Part model, mm, in its own coordinate system. Round coordinates to 2 decimals unless told otherwise and drop trailing zeros. Order: outer loops, then holes, each group sorted by start corner. A loop starts at its lowest first (then second) coordinate and runs counter-clockwise, first axis right, second up. Notation, with made-up numbers: (61, 69.5) -> (71, 69.5) arc R22 ccw to (71, 98.5) -> close; hole circle Ø1 at (-27, 5). An arc over 180 degrees is marked (long way). Answer as a JSON object with one key per item and string values. Group by question number.
Autodesk Inventor part; units mm, degrees
ref_plane "YZ Plane" through (0, 0, 0) normal (1, 0, 0) x (0, 1, 0)
ref_plane "XZ Plane" through (0, 0, 0) normal (0, 1, 0) x (-1, 0, 0)
ref_plane "XY Plane" through (0, 0, 0) normal (0, 0, 1) x (1, 0, 0)
sketch "Skizze1" plane through (0, 0, 0) normal (0, 0, 1) x (1, 0, 0)
  line L0 (-110, -65) -> (110, -65)
  line L1 (110, -65) -> (110, 65)
  line L2 (110, 65) -> (-110, 65)
  line L3 (-110, 65) -> (-110, -65)
  line L4 (-110, -65) -> (110, 65) construction
  line L5 (110, -65) -> (-110, 65) construction
  point P0 (0, 0)
  dimension "d0" = 220
  dimension "d1" = 130
extrude "Grundkörper" add sketch "Skizze1" along normal blind 5
sketch "Skizze2" plane through (0, 0, 5) normal (0, 0, 1) x (1, 0, 0)
  line L0 (110, 65) -> (-110, 65) construction
  line L1 (-110, 65) -> (-110, -65) construction
  line L2 (110, -65) -> (110, 65) construction
  line L3 (-110, -65) -> (110, -65) construction
  line L4 (-95, -50) -> (95, -50) construction
  line L5 (95, -50) -> (95, 50) construction
  line L6 (95, 50) -> (-95, 50) construction
  line L7 (-95, 50) -> (-95, -50) construction
  line L8 (-95, -50) -> (95, 50) construction
  line L9 (95, -50) -> (-95, 50) construction
  line L10 (0, 65) -> (0, -65) construction
  point P0 (0, 0)
  point P1 (0, 50)
  point P2 (-95, 16.6667)
  point P3 (-95, -16.6667)
  point P4 (-95, -50)
  point P5 (0, 50)
  point P6 (0, 16.6667)
  point P7 (0, -16.6667)
  point P8 (0, -50)
  point P9 (-47.5, 50)
  point P10 (-47.5, -50)
  point P11 (0, 50)
  point P12 (0, -50)
  point P13 (95, 50)
  point P14 (95, 16.6667)
  point P15 (95, -16.6667)
  point P16 (95, -50)
  point P17 (95, -50)
  point P18 (47.5, 50)
  point P19 (47.5, -50)
  dimension "d4" = 15
  dimension "d5" = 15
  dimension "d6" = 100
  dimension "d7" = 190
  dimension "d17" = 33.3333
  dimension "d20" = 95
  dimension "d25" = 47.5
hole "Boh_M6" at (-95, 50, 5) at (0, 50, 5) at (-95, 16.6667, 5) at (-95, -16.6667, 5) at (-95, -50, 5) at (-95, -50, 5) at (0, 16.6667, 5) at (0, -16.6667, 5) at (0, -50, 5) at (-47.5, 50, 5) at (-47.5, -50, 5) at (47.5, 50, 5) at (95, 50, 5) at (95, 16.6667, 5) at (95, -16.6667, 5) at (95, -50, 5) at (95, -50, 5) at (47.5, -50, 5) direction (0, 0, -1) diameter 6.6 end through all
equation "\"d0\" = Chassis_Width"
equation "\"Chassis_Width\" = 220"
equation "\"Rocker_Screw_Distance\" = 32.5"
equation "\"Rocker_Screw_Distance_Bottom\" = 76"
properties part number "100-10-FRAME-DIFFERENTIAL-REINF-01" material "Aluminium 6061"
Q1. Band-saw the part on A-A (x = -95). List the corners of the cut face in (y, z), plus the area to 3 significant figures.
Q2. Wall check: line 1 (X direction, y = -50, z = 2.45); line 2 (Y direction, x = -47.5, z = 3.2); line 3 (Y direction, x = -95, z = 1.25). Give the ranges that are in metal, low to high. Write a range as [from, to].
Q3. Two-plate mould, pull along Y, no slides. Class faces 1 (the flat face through (-2, -65, 2)), 2 (the flat face through (-2, 1, 5)), 3 (the cylindrical face through (-97.23, 52.43, 2.46)): +Y half, -Y half, draft (parallel to the pull), parting line (faces both ways), or undercut.
Q4. Band-saw the part on D-D (x = 47.5). List the corners of the cut face in (y, z), plus the area to 3 significant figures.
Q5. Band-saw the part on B-B (z = 3.85). Count the separate pieces of the cut face and the enclosed holes in it, plus the area to 3 significant figures.
Q6. Band-saw the part on C-C (y = 50). List the corners of the cut face in (x, z).
Completed:
{
 "1": {"outline": "(-65, 0) -> (-53.3, 0) -> (-53.3, 5) -> (-65, 5) -> close; (-46.7, 0) -> (-19.97, 0) -> (-19.97, 5) -> (-46.7, 5) -> close; (-13.37, 0) -> (13.37, 0) -> (13.37, 5) -> (-13.37, 5) -> close; (19.97, 0) -> (46.7, 0) -> (46.7, 5) -> (19.97, 5) -> close; (53.3, 0) -> (65, 0) -> (65, 5) -> (53.3, 5) -> close", "area": "518 mm2"},
 "2": {"line 1": "[-110, -98.3], [-91.7, -50.8], [-44.2, -3.3], [3.3, 44.2], [50.8, 91.7], [98.3, 110]", "line 2": "[-65, -53.3], [-46.7, 46.7], [53.3, 65]", "line 3": "[-65, -53.3], [-46.7, -19.97], [-13.37, 13.37], [19.97, 46.7], [53.3, 65]"},
 "3": {"face 1": "-Y half", "face 2": "draft", "face 3": "undercut"},
 "4": {"outline": "(-65, 0) -> (-53.3, 0) -> (-53.3, 5) -> (-65, 5) -> close; (-46.7, 0) -> (46.7, 0) -> (46.7, 5) -> (-46.7, 5) -> close; (53.3, 0) -> (65, 0) -> (65, 5) -> (53.3, 5) -> close", "area": "584 mm2"},
 "5": {"separate pieces": "1", "enclosed holes": "16", "area": "28,100 mm2"},
 "6": {"outline": "(-110, 0) -> (-98.3, 0) -> (-98.3, 5) -> (-110, 5) -> close; (-91.7, 0) -> (-50.8, 0) -> (-50.8, 5) -> (-91.7, 5) -> close; (-44.2, 0) -> (-3.3, 0) -> (-3.3, 5) -> (-44.2, 5) -> close; (3.3, 0) -> (44.2, 0) -> (44.2, 5) -> (3.3, 5) -> close; (50.8, 0) -> (91.7, 0) -> (91.7, 5) -> (50.8, 5) -> close; (98.3, 0) -> (110, 0) -> (110, 5) -> (98.3, 5) -> close"}
}
